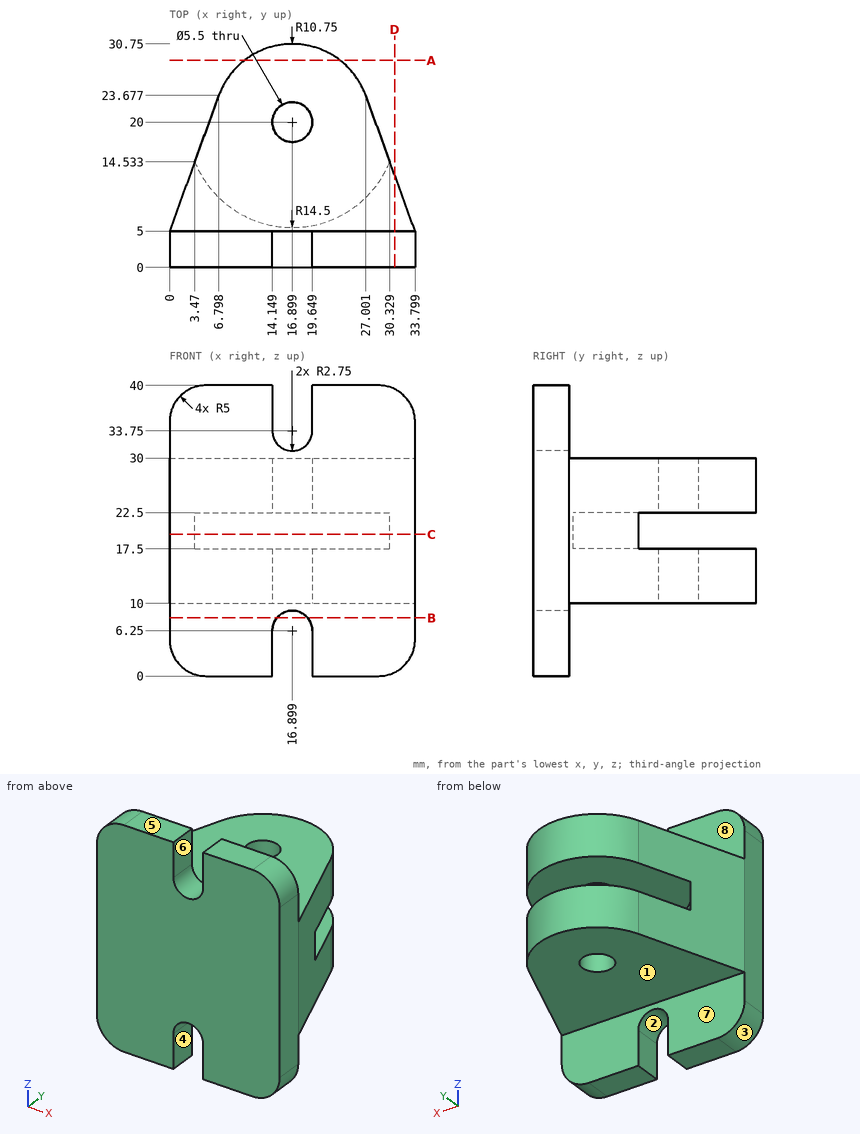
Can you work these out from the drawing? Everything is in mm from the part's minimum corner. A direction names the side the tool comes from. Give positions to 0.01 mm unless a question says otherwise; leave off trailing zeros. Loops run counter-clockwise (first coordinate to the right, second up) from the corner with the lowest first, then second, coordinate; pieces in that order, holes last. Notation, with made-up numbers: (-24, 68) -> (32, 68) arc R10 cw to (32, 78) -> close; hole circle Ø1 at (68, -39). An arc over 180 degrees is marked (long way). Put each result on its own line as item: value.
(1) Imagine slicing it at B-B on z = 8. Write out the boundary of the cut face in (x, y), plus the area to 3 significant figures.
Computed:
outline: (0, 0) -> (14.78, 0) -> (14.78, 5) -> (0, 5) -> close; (19.02, 0) -> (33.8, 0) -> (33.8, 5) -> (19.02, 5) -> close
area: 148 mm^2
(2) Imagine slicing it at A-A on y = 28.5. Write out the boundary of the cut face in (x, z).
Computed:
outline: (10.32, 10) -> (23.48, 10) -> (23.48, 17.5) -> (10.32, 17.5) -> close; (10.32, 22.5) -> (23.48, 22.5) -> (23.48, 30) -> (10.32, 30) -> close
(3) I'm going to push flat-ended pins straight in: pin 1 Ø3 at (x, y) = (29.5, 10.5) entering from -Z; pin 2 Ø6 at (y, z) = (17.5, 25) entering from -X; pin 3 Ø4 at (y, z) = (2.5, 38) entering from +X; pin 4 Ø3.5 at (x, y) = (16.9, 20) entering from +Z. Where does each tip first touch, or does it pass through?
Computed:
pin 1: z = 10
pin 2: x = 3.46
pin 3: x = 33.7
pin 4: through
(4) Please list where these lines run through material, in increasing order: probe 1 along Z at (x, y) = (14, 24); probe 2 along Y at (x, z) = (4, 36); probe 3 along Z at (x, y) = (26.5, 6). Write a range as [from, to].
Computed:
probe 1: [10, 17.5], [22.5, 30]
probe 2: [0, 5]
probe 3: [10, 30]
(5) Thinking about a two-plate mould opening in X: for the marked faces 1, 2 and 3, which applies, pulls with the +X half, pulls with the -X half, needs draft (parallel to the pull), parting line crosses it, or undercut?
Computed:
face 1: needs draft
face 2: undercut
face 3: pulls with the -X half
(6) For the marked faces 4, 5, 6, 7 and 8, which set-ups out of +Z, -Z, +X, -X, +Y, -Y let a thin tool reach every point of the face, with its end or its side?
Computed:
face 4: -Z, +Y, -Y
face 5: +Z, +X, -X, +Y, -Y
face 6: +Z, +Y, -Y
face 7: -Z, +X, -X, +Y
face 8: +Z, +X, -X, +Y
(7) Imagine slicing it at D-D on x = 31. Write out the boundary of the cut face in (y, z).
Computed:
outline: (0, 0.51) -> (5, 0.51) -> (5, 10) -> (12.69, 10) -> (12.69, 30) -> (5, 30) -> (5, 39.49) -> (0, 39.49) -> close
(8) Imagine slicing it at C-C on z = 19.5. Write out the boundary of the cut face in (x, y).
Computed:
outline: (0, 0) -> (33.8, 0) -> (33.8, 5) -> (30.33, 14.53) arc R14.5 cw to (3.47, 14.53) -> (0, 5) -> close
